Job drawing, mm, ordinate dimensions from the low corner. One solid piece. A direction names the side the tool comes from. Give positions to 0.01 mm unless a question says otherwise; leave off trailing zeros. Loops run counter-clockwise (first coordinate to the right, second up) from the corner with the lowest first, then second, coordinate; pieces in that order, holes last. Notation, with made-up numbers: (57.5, 69) -> (83.5, 69) arc R19 cw to (83.5, 100) -> close; hole circle Ø3 at (31.5, 37.5). An arc over 180 degrees is marked (long way). Use one line per item in the form item = value.
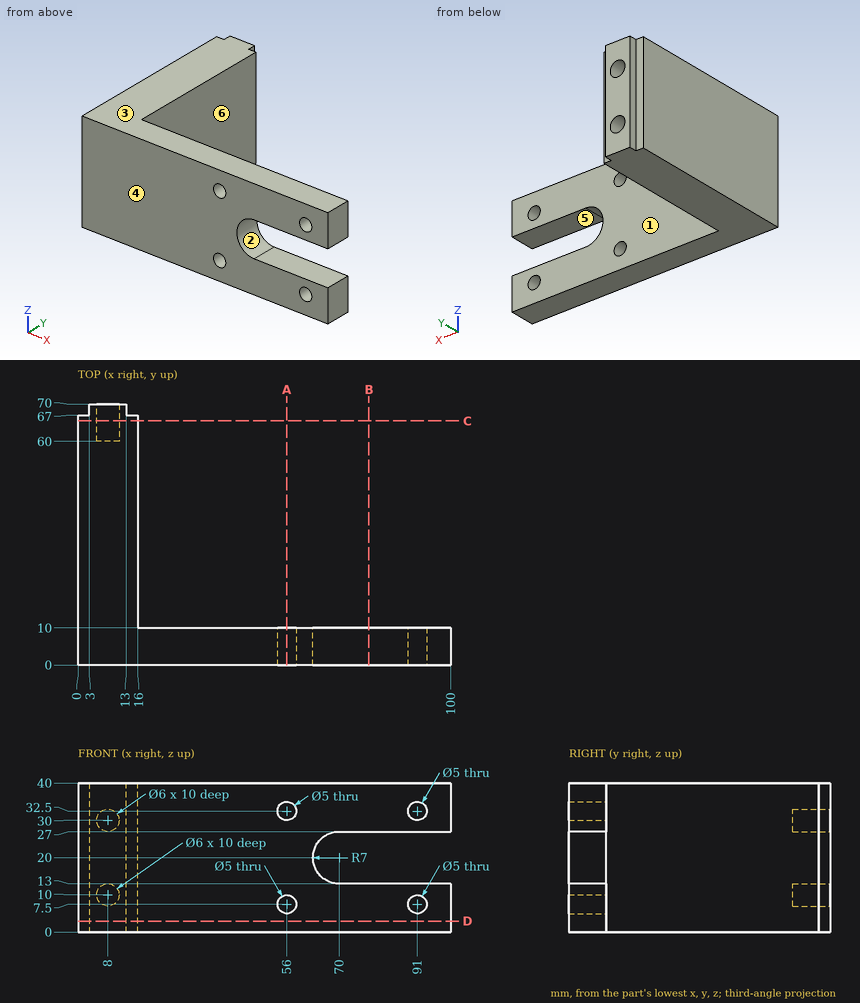
1. Cut at D-D, the plane z = 3. Write the cut outline in (x, y).
Result sheet:
outline = (0, 0) -> (100, 0) -> (100, 10) -> (16, 10) -> (16, 67) -> (13, 67) -> (13, 70) -> (3, 70) -> (3, 67) -> (0, 67) -> close
2. Cut at A-A, the plane x = 56. Write the cut outline in (y, z), then the cut area to 3 significant figures.
Result sheet:
outline = (0, 0) -> (10, 0) -> (10, 5) -> (0, 5) -> close; (0, 10) -> (10, 10) -> (10, 30) -> (0, 30) -> close; (0, 35) -> (10, 35) -> (10, 40) -> (0, 40) -> close
area = 300 mm^2
3. Drop flat-ended pins along their axis: P1, Ø3, axis at x = 8, z = 29, coming from the +Y side; P2, Ø2.5, axis at y = 69, z = 20, coming from the -X side; P3, Ø1, axis at x = 38.5, z = 36, coming from the +Y side. Give the stop position or say it passes through.
Result sheet:
P1 = 60
P2 = 3
P3 = 10
4. Cut at C-C, the plane y = 65.5. Write the cut outline in (x, z), then the cut area to 3 significant figures.
Result sheet:
outline = (0, 0) -> (16, 0) -> (16, 40) -> (0, 40) -> close; hole circle Ø6 at (8, 10); hole circle Ø6 at (8, 30)
area = 583 mm^2
5. Drill centre lines: line 1 (Z direction, x = 91, y = 2); line 2 (Z direction, x = 8, y = 64.75); line 3 (X direction, y = 3.75, z = 32.5). Where is each one in solid material? Low to high.
Result sheet:
line_1 = 0 to 5, 10 to 13, 27 to 30, 35 to 40
line_2 = 0 to 7, 13 to 27, 33 to 40
line_3 = 0 to 53.5, 58.5 to 88.5, 93.5 to 100
6. Mould opens along Z. For the marked faces 1, 2 and 3 say: pulls with the +Z half, pulls with the -Z half, needs draft (parallel to the pull), parting line crosses it, or undercut.
Result sheet:
face_1 = needs draft
face_2 = undercut
face_3 = pulls with the +Z half
7. Cut at B-B, the plane x = 78. Write the cut outline in (y, z), then the cut area to 3 significant figures.
Result sheet:
outline = (0, 0) -> (10, 0) -> (10, 13) -> (0, 13) -> close; (0, 27) -> (10, 27) -> (10, 40) -> (0, 40) -> close
area = 260 mm^2
8. Tool access for the marked faces 4, 5 and 6: list every direction of +Z, -Z, +X, -X, +Y, -Y with a clear straight run to the whole face (end or side of a thin tool).
Result sheet:
face_4 = +Z, -Z, +X, -X, -Y
face_5 = +X, +Y, -Y
face_6 = +Z, -Z, +X, +Y
